```python
from build123d import *

# Parameters (mm, degrees)
F0_R     = 3.81
F3_R     = 3.81
F4_DEPTH = 6.35
F7_R     = 3.81
F8_DEPTH = 6.35


with BuildPart() as f2:
    # F2: sweep along a path in F1
    with BuildLine(Plane.XY) as f2_path:
        ThreePointArc((0, 0), (2.5964520368, -19.7220112368), (10.2088642316, -38.1))
    # F0 (on Front) → F2 (sweep)
    with BuildSketch(Plane.XZ):
        Circle(F0_R)
    sweep(path=f2_path.line)

    # F3 (on Right) → F4 (join, symmetric)
    with BuildSketch(Plane.YZ):
        Circle(F3_R)
    extrude(amount=F4_DEPTH, both=True)

    # F7 (on face) → F8 (join, symmetric)
    with BuildSketch(Plane(origin=(-8.8411357684, -5.1044321158, 0), x_dir=(-0.5, 0.8660254038, 0), z_dir=(0.8660254038, 0.5, 0))):
        with Locations((-38.1, 0)):
            Circle(F7_R)
    extrude(amount=F8_DEPTH, both=True)


solid = f2.part
```
CAD build for the part. Positions are in the model's coordinates, mm. A direction names the side the tool comes from. Give positions to 0.01 mm unless a question says otherwise; leave off trailing zeros. Order: outer loops, then holes, each group sorted by start corner. A loop starts at its lowest first (then second) coordinate and runs counter-clockwise, first axis right, second up. Notation, with made-up numbers: M 11,16.25 L 17,16.25 A27 ccw 17,35.25 Z; hole C 77.25,49.25 d2. An arc over 180 degrees is marked long. Put each result on its own line as item: value. Start each with the question number.
(1) Saw through at B-B, the plane z = -3. Write the cut outline in (x, y).
(2) Mould opens along X. For faces 1 (the flat face through (6.35, 0, 0)), 2 (the cylindrical face through (12.19, -41.35, 0.17)), 3 (the flat face through (-6.35, 0, 0)) say: +X half, -X half, draft (parallel to the pull), parting line (faces both ways), or undercut.
(3) Saw through at A-A, the plane z = 0. Write the cut outline in (x, y), then the cut area to 3 significant figures.
(4) Flat gauge pins, fed straight in: pin 1 Ø4 at (y, z) = (-0.5, -0.5) entering from +X; pin 2 Ø3 at (y, z) = (-21, -1) entering from +X; pin 3 Ø1.5 at (x, z) = (-3.5, 1) entering from +Y. Where does each tip first touch, or does it go through?
(5) Drill centre lines: line 1 along X through (y, z) = (2, -1.25); line 2 along X through (y, z) = (-32.5, -1.5); line 3 along Z through (x, y) = (11, -36). Where is each one in solid material? Low to high.
(6) Which spindle directions (+Z, -Z, +X, -X, +Y, -Y) get a long thin tool onto all of the face, cutting with end or side? Do faces 4 (the cylindrical face through (0.089, 3.634, 1.144)), 5 (the flat face through (4.736, -41.321, 0.053)). Say none if no direction does.
Check result:
1. outline: M -6.35,-2.35 L -2.31,-2.35 A78.55 ccw 7.03,-37.22 L 3.54,-39.24 L 5.88,-43.31 L 16.88,-36.96 L 14.53,-32.89 L 11.1,-34.87 A73.85 cw 2.39,-2.35 L 6.35,-2.35 L 6.35,2.35 L -6.35,2.35 Z
2. face 1: +X half
2. face 2: undercut
2. face 3: -X half
3. outline: M -6.35,-3.81 L -3.72,-3.81 A80.01 ccw 5.08,-36.66 L 2.8,-37.98 L 6.61,-44.57 L 17.61,-38.22 L 13.8,-31.63 L 11.69,-32.85 A72.39 cw 3.91,-3.81 L 6.35,-3.81 L 6.35,3.81 L -6.35,3.81 Z
3. area: 439 mm2
4. pin 1: stops at x = 6.35
4. pin 2: stops at x = 7.33
4. pin 3: stops at y = 3.8
5. line 1: x = -6.35 to 6.35
5. line 2: x = 3.42 to 11.17, 12.9 to 14.31
5. line 3: z = -3.53 to 3.53
6. face 4: none
6. face 5: +Z, -Z, -X, -Y
